Input: part model. Units: mm. Frame: model coordinates. Round coordinates to 2 decimals unless told otherwise and drop trailing zeros. Order: outer loops, then holes, each group sorted by start corner. A loop starts at its lowest first (then second) coordinate and runs counter-clockwise, first axis right, second up. Notation, with made-up numbers: (68, 67) - (115, 67) arc R31 ccw to (115, 102) - close; hole circle Ø1 at (-30, 31.25). An arc over 180 degrees is marked (long way). One line per item, written item: value. Start each with the question number.
Autodesk Inventor part; units mm, degrees
ref_plane "YZ Plane" through (0, 0, 0) normal (1, 0, 0) x (0, 1, 0)
ref_plane "XZ Plane" through (0, 0, 0) normal (0, 1, 0) x (-1, 0, 0)
ref_plane "XY Plane" through (0, 0, 0) normal (0, 0, 1) x (1, 0, 0)
sketch "Sketch1" plane through (0, 0, 0) normal (0, 0, 1) x (1, 0, 0)
  line L0 (60.0759, 197.5616) -> (45.0759, 197.5616)
  line L1 (45.0759, 197.5616) -> (45.0759, 200.5616)
  line L2 (15.0759, 200.5616) -> (15.0759, 197.5616)
  line L3 (45.0759, 200.5616) -> (15.0759, 200.5616)
  line L4 (15.0759, 197.5616) -> (0.0759, 197.5616)
  line L5 (57.0759, 81.5616) -> (60, 81.5616)
  line L6 (0.0759, 77.6616) -> (-2.9241, 77.6616)
  line L7 (-2.9241, 77.6616) -> (-2.9241, 47.8616)
  line L8 (-2.9241, 47.8616) -> (0.0759, 47.8616)
  line L9 (60, 4.5616) -> (60, 81.5616)
  line L10 (0.0759, 47.8616) -> (0.0759, 4.5616)
  line L11 (0.0759, 4.5616) -> (15.0759, 4.5616)
  line L12 (60.0757, 4.4159) -> (60, 4.5616)
  line L13 (45.0759, 4.4159) -> (60.0757, 4.4159)
  line L14 (45.0759, 4.4159) -> (45.0759, 1.4159)
  line L15 (45.0759, 1.4159) -> (15.0759, 1.5616)
  line L16 (15.0759, 1.5616) -> (15.0759, 4.5616)
  line L17 (0.0759, 197.5616) -> (0.0759, 154.2616)
  line L18 (0.0759, 154.2616) -> (-2.9241, 154.2616)
  line L19 (60.0759, 121.5616) -> (60.0759, 197.5616)
  line L20 (60.0759, 121.5616) -> (57.0759, 121.5616)
  line L21 (-2.9241, 124.2616) -> (0.0759, 124.2616)
  line L22 (-2.9241, 154.2616) -> (-2.9241, 124.2616)
  line L23 (0.0759, 124.2616) -> (0.0759, 77.6616)
  line L24 (57.0759, 121.5616) -> (57.0759, 81.5616)
  point P0 (0, 0)
  dimension "d47" = 193
  dimension "d48" = 60
  dimension "d49" = 3
  dimension "d50" = 30
  dimension "d51" = 15
  dimension "d52" = 3
  dimension "d53" = 3
  dimension "d54" = 15
  dimension "d55" = 3
  dimension "d56" = 3
  dimension "d57" = 3
  dimension "d58" = 3
  dimension "d59" = 15
  dimension "d60" = 40
  dimension "d61" = 3
  dimension "d62" = 77
  dimension "d63" = 3
  dimension "d64" = 76
  dimension "d65" = 199.1457
  dimension "d66" = 43.3
  dimension "d67" = 46.6
  dimension "d68" = 43.3
  dimension "d69" = 30
  dimension "d70" = 29.8
extrude "Extrusion1" add sketch "Sketch1" along normal blind 3
properties part number "sampingkiri"
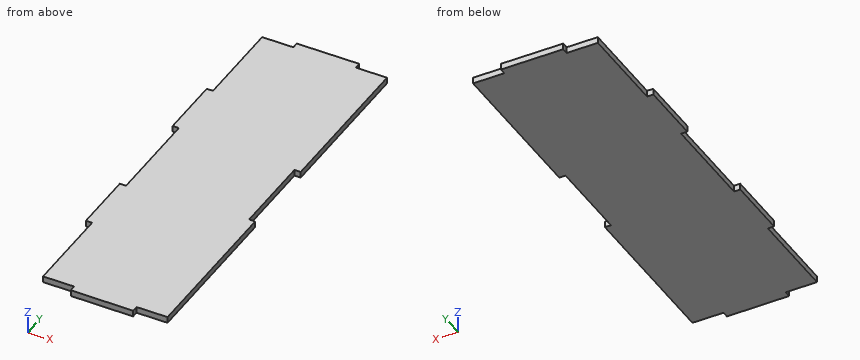
Item 1: Section query C-C on y = 157.5. Return loops of the section in (x, z).
Item 2: First-contact query: pin 1 Ø0.9 at (y, z) = (94.5, 2) entering from -X; pin 2 Ø1 at (x, z) = (34.5, 2.5) entering from -Y; pin 3 Ø1.5 at (x, z) = (-1.5, 1) entering from +Y. Flat tips, straight axial feed; report the tip coordinate or a pass-through.
Item 3: Line query: L1, parallel to X at y = 55.5, z = 1.25; L2, parallel to Y at x = 20, z = 0.55; L3, parallel to X at y = 111, z = 0.2. Output: solid intervals per line, ascending.
Item 4: Section query B-B on x = 54.5. Return loops of the section in (y, z).
Item 5: Section query A-A on z = 1.4. Return loops of the section in (x, y).
Geometry results:
1. outline: (0.08, 0) - (60.08, 0) - (60.08, 3) - (0.08, 3) - close
2. pin 1: stops at x = 0.08
2. pin 2: stops at y = 1.46
2. pin 3: stops at y = 154.26
3. L1: x = -2.92 to 60
3. L2: y = 1.54 to 200.56
3. L3: x = 0.08 to 57.08
4. outline: (4.42, 0) - (197.56, 0) - (197.56, 3) - (4.42, 3) - close
5. outline: (-2.92, 47.86) - (0.08, 47.86) - (0.08, 4.56) - (15.08, 4.56) - (15.08, 1.56) - (45.08, 1.42) - (45.08, 4.42) - (60.08, 4.42) - (60, 4.56) - (60, 81.56) - (57.08, 81.56) - (57.08, 121.56) - (60.08, 121.56) - (60.08, 197.56) - (45.08, 197.56) - (45.08, 200.56) - (15.08, 200.56) - (15.08, 197.56) - (0.08, 197.56) - (0.08, 154.26) - (-2.92, 154.26) - (-2.92, 124.26) - (0.08, 124.26) - (0.08, 77.66) - (-2.92, 77.66) - close
